from build123d import *

# Parameters (mm, degrees)
BOSS_EXTRUDE1_DEPTH = 62.70625
CUT_EXTRUDE1_DEPTH  = 224.410663511
SKETCH3_R           = 1.625
SKETCH3_R_2         = 3.175
CUT_EXTRUDE2_DEPTH  = 224.410663511


with BuildPart() as part:
    # Sketch1 → Boss-Extrude1 (new, symmetric)
    with BuildSketch(Plane.XY):
        with BuildLine():
            Line((-9.525, 149.225), (-4.7625, 149.225))
            Line((-4.7625, 149.225), (-4.7625, 0))
            ThreePointArc((-4.7625, 0), (-3.367596045, -3.367596045), (0, -4.7625))
            Line((0, -4.7625), (149.225, -4.7625))
            Line((149.225, -4.7625), (149.225, -9.525))
            Line((149.225, -9.525), (0, -9.525))
            ThreePointArc((0, -9.525), (-6.735192091, -6.735192091), (-9.525, 0))
            Line((-9.525, 0), (-9.525, 149.225))
        make_face()
    extrude(amount=BOSS_EXTRUDE1_DEPTH, both=True)

    # Sketch2 → Cut-Extrude1 (cut, through all)
    with BuildSketch(Plane(origin=(-4.7625, 0, 0), x_dir=(0, 0, -1), z_dir=(1, 0, 0))):
        with BuildLine():
            Line((-50.8, 134.9375), (-50.8, 128.5875))
            ThreePointArc((-50.8, 128.5875), (-44.45, 122.2375), (-38.1, 128.5875))
            Line((-38.1, 128.5875), (-38.1, 134.9375))
            ThreePointArc((-38.1, 134.9375), (-44.45, 141.2875), (-50.8, 134.9375))
        make_face()
        with BuildLine():
            Line((-50.8, 46.0375), (-50.8, 39.6875))
            ThreePointArc((-50.8, 39.6875), (-44.45, 33.3375), (-38.1, 39.6875))
            Line((-38.1, 39.6875), (-38.1, 46.0375))
            ThreePointArc((-38.1, 46.0375), (-44.45, 52.3875), (-50.8, 46.0375))
        make_face()
        with BuildLine():
            Line((38.1, 39.6875), (38.1, 46.0375))
            ThreePointArc((38.1, 46.0375), (44.45, 52.3875), (50.8, 46.0375))
            Line((50.8, 46.0375), (50.8, 39.6875))
            ThreePointArc((50.8, 39.6875), (44.45, 33.3375), (38.1, 39.6875))
        make_face()
        with BuildLine():
            Line((38.1, 134.9375), (38.1, 128.5875))
            ThreePointArc((38.1, 128.5875), (44.45, 122.2375), (50.8, 128.5875))
            Line((50.8, 128.5875), (50.8, 134.9375))
            ThreePointArc((50.8, 134.9375), (44.45, 141.2875), (38.1, 134.9375))
        make_face()
    cut_extrude1 = extrude(amount=-CUT_EXTRUDE1_DEPTH, mode=Mode.SUBTRACT)

    # Mirror1: Cut-Extrude1 across plane
    add(cut_extrude1.mirror(Plane(origin=(0, 0, 0), x_dir=(0, 0, 1), z_dir=(0.7071067811865475, -0.7071067811865476, 0))), mode=Mode.SUBTRACT)

    # Sketch3 → Cut-Extrude2 (cut, through all)
    with BuildSketch(Plane(origin=(-4.7625, 0, 0), x_dir=(0, 0, -1), z_dir=(1, 0, 0))):
        with Locations((56.35625, 28.575)):
            Circle(SKETCH3_R)
        with Locations((56.35625, 53.975)):
            Circle(SKETCH3_R_2)
    extrude(amount=-CUT_EXTRUDE2_DEPTH, mode=Mode.SUBTRACT)


solid = part.part
The listing builds one solid part. Answer for the finished solid, in the listing's coordinates (mm). A direction names the side the tool comes from. Coordinates: 2 decimals unless noted, no trailing zeros. Write each loop counter-clockwise with the first axis right and the second up, starting at its lowest first coordinate (ties: lowest second). Pieces come first, ordered by that corner, then holes. Notation, with made-up numbers: M -15.5,69.5 L -2.5,69.5 A12 cw -2.5,92.5 Z; hole C -7.75,-23.75 d1. An arc over 180 degrees is marked long. Write each question's results on one line, items separated by ' | '.
Item 1: Which of the six approach directions +Z, -Z, +X, -X, +Y, -Y give full straight-line access (tool end or side, diameter ignored) to faces 4 (the face through (-4.762, 76, 1)), 5 (the face through (122.24, -7.11, -44.31)), 6 (the face through (-7.11, 52.386, 44.31))?
Answer below:
face 4: +Z, -Z, +X, +Y | face 5: +Y, -Y | face 6: +X, -X
Item 2: For a pull along Z with two mould halves and no side action, classify faces 1 (the face through (-3.404, -3.33, 0.878)), 2 (the face through (-7.11, 33.34, 44.59)), 3 (the face through (33.34, -7.11, -44.59)) as released by +Z, released by -Z, zero draft, split by the parting line, or undercut.
Answer below:
face 1: zero draft | face 2: undercut | face 3: undercut
Item 3: Given P1, Ø1, axis at x = 51.5, z = 48.5, coming from the +Y side; P2, Ø4, axis at y = 28.58, z = -56.36, coming from the -X side (3 decimals); P3, Ø1.5, axis at y = 68.5, z = -17.5, coming from the +X side, each flat-ended and moving along its own axis, determine where each tip first touches the part or whether it passes through.
Answer below:
P1: y = -4.76 | P2: x = -9.525 | P3: x = -4.76
Item 4: The part is cut by section B-B on x = 137. Determine the outline of the cut face in (y, z) (1 decimal).
Answer below:
outline: M -9.5,-62.7 L -4.8,-62.7 L -4.8,-50.5 L -9.5,-50.5 Z; M -9.5,-38.4 L -4.8,-38.4 L -4.8,38.4 L -9.5,38.4 Z; M -9.5,50.5 L -4.8,50.5 L -4.8,62.7 L -9.5,62.7 Z
Item 5: The part is cut by section A-A on z = 44.45. State how many separate pieces and enclosed holes the cut face has, and give its area (3 significant figures).
Answer below:
separate pieces: 5 | enclosed holes: 0 | area: 1,110 mm2
Item 6: Consider probe 1 along X at (y, z) = (17, 19) (1 decimal). Determine where the line is inside the solid, lowest interval first. Write a range as [from, to].
Answer below:
probe 1: [-9.5, -4.8]
Item 7: The part is cut by section C-C on y = 36.5. Determine the outline of the cut face in (x, z) (1 decimal).
Answer below:
outline: M -9.5,-62.7 L -4.8,-62.7 L -4.8,-49.9 L -9.5,-49.9 Z; M -9.5,-39 L -4.8,-39 L -4.8,39 L -9.5,39 Z; M -9.5,49.9 L -4.8,49.9 L -4.8,62.7 L -9.5,62.7 Z
